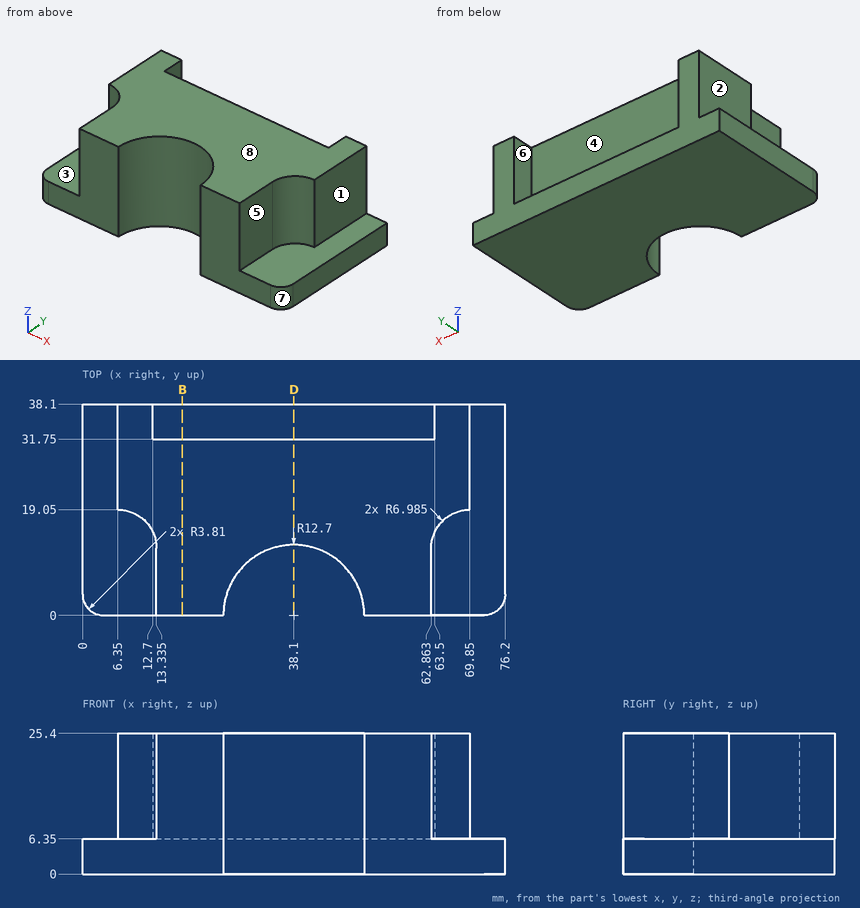
Check sheet for the drawn part. Datum: minimum x, y, z corner. Units: mm. A direction names the side the tool comes from. Round coordinates to 2 decimals unless told otherwise and drop trailing zeros. Order: outer loops, then holes, each group sorted by start corner. A loop starts at its lowest first (then second) coordinate and runs counter-clockwise, first axis right, second up.
(1) Cross-section at D-D, the plane x = 38.1. Enter the section's corners in (y, z), and give its area (3 significant figures).
(2) Cross-section at B-B, the plane x = 18. Enter the section's corners in (y, z), and give its area (3 significant figures).
(3) Draft check along X on the marked faces 6, 7 and 8. Enter one of: pulls with the +X half, pulls with the -X half, needs draft (parallel to the pull), parting line crosses it, or undercut.
(4) Access from +Z, -Z, +X, -X, +Y, -Y to the whole of each face (thin tool, end or side, straight path). Record for the marked faces 1, 2, 3, 4 and 5.
(5) Go/stop test with flat-tipped pins: P1, Ø9.5, axis at x = 27.5, z = 19, coming from the +Y side; P2, Ø3, axis at y = 35, z = 17.5, coming from the +X side; P3, Ø4, axis at x = 3.5, y = 28.5, coming from the +Z side. Record where each tip stops, or that it passes through.
(6) Scan lines: probe 1 along Z at (x, y) = (64, 7.5); probe 2 along X at (y, z) = (30.5, 18.25); probe 3 along X at (y, z) = (10.5, 5) (1 decimal). Record each from-to range of solid material in increasing order.
Check sheet entries:
1. outline: (12.7, 0) - (38.1, 0) - (38.1, 6.35) - (31.75, 6.35) - (31.75, 25.4) - (12.7, 25.4) - close
1. area: 524 mm2
2. outline: (0, 0) - (38.1, 0) - (38.1, 6.35) - (31.75, 6.35) - (31.75, 25.4) - (0, 25.4) - close
2. area: 847 mm2
3. face 6: undercut
3. face 7: pulls with the +X half
3. face 8: needs draft
4. face 1: +Z, +X, +Y, -Y
4. face 2: +Z, -X, +Y, -Y
4. face 3: +Z, -X, -Y
4. face 4: +Z, +Y
4. face 5: +Z, +X, -Y
5. P1: stops at y = 31.75
5. P2: stops at x = 69.85
5. P3: stops at z = 6.35
6. probe 1: z = 0 to 6.35
6. probe 2: x = 6.35 to 69.85
6. probe 3: x = 0 to 31, 45.2 to 76.2
